from build123d import *

# Parameters (mm, degrees)
F0_W     = 61.976
F0_H     = 26.67
F1_DEPTH = 1.5875
F2_R     = 1.016
F2_R_2   = 2.794
F3_DEPTH = 3.175
F4_DEPTH = 12.7
F5_W     = 45.72
F5_H     = 19.05
F6_DEPTH = 6.35


with BuildPart() as f1:
    # F0 (on Top) → F1 (new body)
    with BuildSketch(Plane.XY):
        Rectangle(F0_W, F0_H)
    extrude(amount=F1_DEPTH)

    # F2 (on face) → F3 (join)
    with BuildSketch(Plane.XY.offset(1.5875)):
        with BuildLine():
            ThreePointArc((-25.654, 10.795), (-26.096556, 12.304022), (-27.284026, 13.335))
            Line((-27.284026, 13.335), (-29.611974, 13.335))
            ThreePointArc((-29.611974, 13.335), (-30.423656, 12.770656), (-30.988, 11.958974))
            Line((-30.988, 11.958974), (-30.988, 9.631026))
            ThreePointArc((-30.988, 9.631026), (-27.852317, 8.065238), (-25.654, 10.795))
        make_face()
        with Locations((-28.448, 10.795)):
            Circle(F2_R, mode=Mode.SUBTRACT)
        with Locations((28.448, -10.795)):
            Circle(F2_R_2)
        with Locations((28.448, -10.795)):
            Circle(F2_R, mode=Mode.SUBTRACT)
        with Locations((-28.448, 10.795)):
            Circle(F2_R_2)
        with Locations((-28.448, 10.795)):
            Circle(F2_R, mode=Mode.SUBTRACT)
        with Locations((-28.448, -10.795)):
            Circle(F2_R_2)
        with Locations((-28.448, -10.795)):
            Circle(F2_R, mode=Mode.SUBTRACT)
        with Locations((28.448, 10.795)):
            Circle(F2_R_2)
        with Locations((28.448, 10.795)):
            Circle(F2_R, mode=Mode.SUBTRACT)
        with BuildLine():
            Line((30.988, -11.958974), (30.988, -9.631026))
            ThreePointArc((30.988, -9.631026), (26.472344, -8.819344), (27.284026, -13.335))
            Line((27.284026, -13.335), (29.611974, -13.335))
            ThreePointArc((29.611974, -13.335), (30.423656, -12.770656), (30.988, -11.958974))
        make_face()
        with Locations((28.448, -10.795)):
            Circle(F2_R, mode=Mode.SUBTRACT)
    extrude(amount=F3_DEPTH)

    # F2 (on face) → F4 (cut)
    with BuildSketch(Plane.XY.offset(1.5875)):
        with Locations((-28.448, 10.795)):
            Circle(F2_R)
        with Locations((28.448, -10.795)):
            Circle(F2_R)
        with Locations((28.448, 10.795)):
            Circle(F2_R)
        with Locations((-28.448, -10.795)):
            Circle(F2_R)
    extrude(amount=-F4_DEPTH, mode=Mode.SUBTRACT)

    # F5 (on face) → F6 (cut)
    with BuildSketch(Plane.XY.offset(1.5875)):
        Rectangle(F5_W, F5_H)
    extrude(amount=-F6_DEPTH, mode=Mode.SUBTRACT)


solid = f1.part
Part model, mm, in its own coordinate system. A direction names the side the tool comes from. Round coordinates to 2 decimals unless told otherwise and drop trailing zeros. Write each loop counter-clockwise with the first axis right and the second up, starting at its lowest first coordinate (ties: lowest second). Pieces come first, ordered by that corner, then holes. Notation, with made-up numbers: M 62,42.25 L 89,42.25 A15 cw 89,58.25 Z; hole C 5.5,15 d3. An arc over 180 degrees is marked long. Return JSON: item names as keys, results as strings. Group by question number.
(1) Pin check, flat tips, straight feed: pin 1 Ø5 at (x, y) = (-20, 8) entering from +Z; pin 2 Ø1.8 at (x, y) = (-28.448, -10.795) entering from +Z; pin 3 Ø1.5 at (x, z) = (-4, 1) entering from -Y (3 decimals); pin 4 Ø0.8 at (y, z) = (-4, 0.5) entering from -X. Stop position of each tip, or through.
(2) Saw through at C-C on z = 3.5. Write the cut outline in (x, y) (3 decimals).
(3) Saw through at B-B on x = 9. Write the cut outline in (y, z) (1 decimal).
(4) Two-plate mould, pull along X, no slides. Class faces 4 (the face through (0, 12, 0)), 5 (the face through (30.988, 0, 1)), 6 (the face through (-30.988, 0, 1)), 7 (the face through (0, -9.525, 1)): +X half, -X half, draft (parallel to the pull), parting line (faces both ways), or undercut.
(5) Which spindle directions (+Z, -Z, +X, -X, +Y, -Y) get a long thin tool onto all of the face, cutting with end or side? Do faces 1 (the face through (-26.946, -8.439, 3.153)), 2 (the face through (-22.86, 0, 1)), 3 (the face through (30.6, -12.9, 1.588)). Say none if no direction does.
(6) Saw through at A-A on y = -2. Write the cut outline in (x, z).
(7) Drill centre lines: probe 1 along Y at (x, z) = (28.5, 1.35) (3 decimals); probe 2 along Y at (x, z) = (1.5, 1.3) (3 decimals); probe 3 along X at (y, z) = (-10.75, 0.9). Where is each one in solid material? Low to high.
(8) Saw through at D-D on x = 23.5. Write the cut outline in (y, z) (1 decimal).
Returned:
{
 "1": {"pin 1": "z = 1.59", "pin 2": "through", "pin 3": "y = -13.335", "pin 4": "x = -30.99"},
 "2": {"outline": "C -28.448,-10.795 d5.588; M -30.988,11.959 A2.794 ccw long -29.612,13.335 A2.794 ccw Z; C 28.448,10.795 d5.588; M 29.612,-13.335 A2.794 ccw 30.988,-11.959 A2.794 ccw long Z; hole C -28.448,-10.795 d2.032; hole C -28.448,10.795 d2.032; hole C 28.448,-10.795 d2.032; hole C 28.448,10.795 d2.032"},
 "3": {"outline": "M -13.3,0 L -9.5,0 L -9.5,1.6 L -13.3,1.6 Z; M 9.5,0 L 13.3,0 L 13.3,1.6 L 9.5,1.6 Z"},
 "4": {"face 4": "draft", "face 5": "+X half", "face 6": "-X half", "face 7": "undercut"},
 "5": {"face 1": "+Z", "face 2": "+Z, -Z", "face 3": "+Z, +X, -Y"},
 "6": {"outline": "M -30.99,0 L -22.86,0 L -22.86,1.59 L -30.99,1.59 Z; M 22.86,0 L 30.99,0 L 30.99,1.59 L 22.86,1.59 Z"},
 "7": {"probe 1": "-13.335 to -11.81, -9.78 to 9.78, 11.81 to 13.335", "probe 2": "-13.335 to -9.525, 9.525 to 13.335", "probe 3": "-30.99 to -29.46, -27.43 to 27.43, 29.46 to 30.99"},
 "8": {"outline": "M -13.3,0 L 13.3,0 L 13.3,1.6 L -13.3,1.6 Z"}
}
